Here's how the part is built. I have some questions about the finished solid (model axes, mm). Round coordinates to 2 decimals unless told otherwise and drop trailing zeros. Loops run counter-clockwise (first coordinate to the right, second up) from the corner with the lowest first, then second, coordinate; pieces in that order, holes last. Notation, with made-up numbers: (51.5, 1) -> (78.5, 1) arc R26 ccw to (78.5, 27) -> close; hole circle Ø3 at (81.5, 86.25). An arc over 180 degrees is marked (long way). Use CSV: the item, a comma, the result in double quotes. Start each with the question number.
from build123d import *

# Parameters (mm, degrees)
F0_W           = 69.9042
F0_H           = 48.707396
F1_DEPTH       = 25
F2_R           = 5
F4_D           = 5
F4_CBORE_D     = 10
F4_CBORE_DEPTH = 5


with BuildPart() as f1:
    # F0 (on Top) → F1 (new body)
    with BuildSketch(Plane.XY):
        Rectangle(F0_W, F0_H)
    extrude(amount=F1_DEPTH)

    # F2
    f2_edges = [f1.edges().sort_by_distance(p)[0] for p in [
        (0, 24.353698, 25),
        (34.9521, 0, 25),
        (0, -24.353698, 25),
        (-34.9521, 0, 25),
        (0, -24.353698, 0),
        (34.9521, 0, 0),
    ]]
    fillet(f2_edges, radius=F2_R)

    # F4 (through all)
    with Locations(Plane.XZ.offset(24.353698)):
        with Locations((0, 13.67986)):
            CounterBoreHole(F4_D / 2, F4_CBORE_D / 2, F4_CBORE_DEPTH)


solid = f1.part
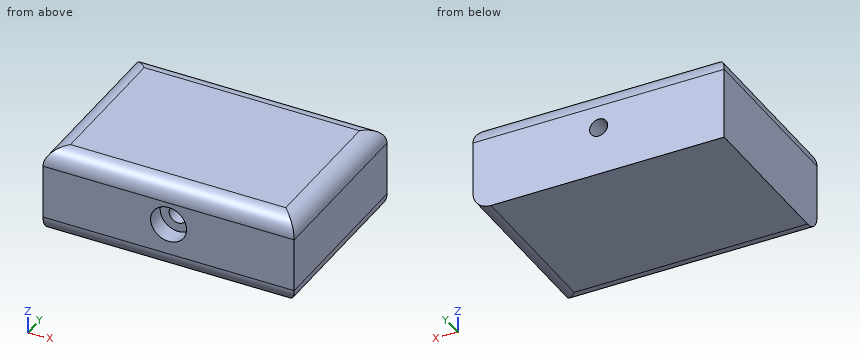
Q1. I want a section at C-C, the plane y = 3. List the corners of the cut face in (x, z) for me.
Q2. I want a section at A-A, the plane x = 0. List the corners of the cut face in (y, z) for me, then the cut area to 3 significant figures.
Q3. I need wall thicknesses on line 1 along Z through (x, y) = (0, -6); line 2 along X through (y, z) = (-9, 13.75); line 3 along Y through (x, z) = (-3, 14). Which ranges of each line are inside material? Lowest first, please.
Q4. Will these pins go through, and if not, where does the flat tip stop? pin 1 Ø4.5 at (x, z) = (0, 13.68) entering from -Y; pin 2 Ø1 at (y, z) = (-19.5, 3.5) entering from +X; pin 3 Ø3 at (x, z) = (-1.5, 13) entering from -Y.
Q5. I want a section at B-B, the plane y = -20.5. List the corners of the cut face in (x, z) for me, then the cut area to 3 significant figures.
Values found:
1,outline,"(-34.95, 0) -> (29.95, 0) arc R5 ccw to (34.95, 5) -> (34.95, 20) arc R5 ccw to (29.95, 25) -> (-29.95, 25) arc R5 ccw to (-34.95, 20) -> close; hole circle Ø5 at (0, 13.68)"
2,outline,"(-24.35, 5) arc R5 ccw to (-19.35, 0) -> (24.35, 0) -> (24.35, 11.18) -> (-19.35, 11.18) -> (-19.35, 8.68) -> (-24.35, 8.68) -> close; (-24.35, 18.68) -> (-19.35, 18.68) -> (-19.35, 16.18) -> (24.35, 16.18) -> (24.35, 20) arc R5 ccw to (19.35, 25) -> (-19.35, 25) arc R5 ccw to (-24.35, 20) -> close"
2,area,"933 mm2"
3,line 1,"0 to 11.18, 16.18 to 25"
3,line 2,"-34.95 to -2.5, 2.5 to 34.95"
3,line 3,"-19.35 to 24.35"
4,pin 1,"through"
4,pin 2,"x = 34.85"
4,pin 3,"y = -19.35"
5,outline,"(-34.95, 0.13) -> (31.1, 0.13) arc R5 ccw to (34.95, 5) -> (34.95, 20) arc R5 ccw to (31.1, 24.87) -> (-31.1, 24.87) arc R5 ccw to (-34.95, 20) -> close; hole circle Ø10 at (0, 13.68)"
5,area,"1,640 mm2"
